Verification items for the finished model (mm, model axes). A direction names the side the tool comes from. Coordinates: 2 decimals unless noted, no trailing zeros. Order: outer loops, then holes, each group sorted by start corner. A loop starts at its lowest first (then second) coordinate and runs counter-clockwise, first axis right, second up. Notation, with made-up numbers: M 66,-34 L 94,-34 A23 ccw 94,-11 Z; hole C 5.5,-16 d11. An arc over 180 degrees is marked long. Return JSON: item names as keys, results as strings. Group by question number.
1. Section check D-D, the plane z = -4. Record the cut outline in (x, y).
2. Section check A-A, the plane y = 0.1. Record the cut outline in (x, z), plus the area to 3 significant figures.
3. Mould release check, pull along X, two halves, no side actions. Record for faces 1 (the flat face through (-45, 0, 9.5)), 2 (the flat face through (0, 0, 3)), 3 (the flat face through (-57.5, 0, 0)): +X half, -X half, draft (parallel to the pull), parting line (faces both ways), or undercut.
4. Section check C-C, the plane x = -6. Record the cut outline in (y, z).
5. Section check B-B, the plane z = 7.25. Record the cut outline in (x, y).
6. Material ranges on line 1 along X through (y, z) = (1.4, 5.75); line 2 along X through (y, z) = (-0.65, -6.5); line 3 along Z through (x, y) = (-10.5, 0.65), recorded low to high.
7. Set-up check for faces 4 (the cylindrical face through (25.617, -0.028, -8.294)), 5 (the cylindrical face through (-25.617, -0.028, 8.294)), 6 (the flat face through (-45, 0, -9.5)): record each of +Z, -Z, +X, -X, +Y, -Y from which the full face is reachable in a straight line by a thin tool's end or side.
```python
from build123d import *

# Parameters (mm, degrees)
F1_DEPTH = 2


with BuildPart() as f1:
    # F0 (on Front) → F1 (new body, symmetric)
    with BuildSketch(Plane.XZ):
        with BuildLine():
            Line((11.751494, 3), (0, 3))
            Line((0, 3), (-11.751494, 3))
            ThreePointArc((-11.751494, 3), (-15.797231, 3.597313), (-19.497744, 5.338285))
            ThreePointArc((-19.497744, 5.338285), (-25.709291, 8.323868), (-32.5, 9.5))
            Line((-32.5, 9.5), (-57.5, 9.5))
            Line((-57.5, 9.5), (-57.5, -9.5))
            Line((-57.5, -9.5), (-32.5, -9.5))
            ThreePointArc((-32.5, -9.5), (-25.709291, -8.323868), (-19.497744, -5.338285))
            ThreePointArc((-19.497744, -5.338285), (-15.797231, -3.597313), (-11.751494, -3))
            Line((-11.751494, -3), (0, -3))
            Line((0, -3), (11.751494, -3))
            ThreePointArc((11.751494, -3), (15.797231, -3.597313), (19.497744, -5.338285))
            ThreePointArc((19.497744, -5.338285), (25.709291, -8.323868), (32.5, -9.5))
            Line((32.5, -9.5), (57.5, -9.5))
            Line((57.5, -9.5), (57.5, 9.5))
            Line((57.5, 9.5), (32.5, 9.5))
            ThreePointArc((32.5, 9.5), (25.709291, 8.323868), (19.497744, 5.338285))
            ThreePointArc((19.497744, 5.338285), (15.797231, 3.597313), (11.751494, 3))
        make_face()
    extrude(amount=F1_DEPTH, both=True)


solid = f1.part
```
Answers follow:
{
 "1": {"outline": "M -57.5,-2 L -16.95,-2 L -16.95,2 L -57.5,2 Z; M 16.95,-2 L 57.5,-2 L 57.5,2 L 16.95,2 Z"},
 "2": {"outline": "M -57.5,-9.5 L -32.5,-9.5 A25 ccw -19.5,-5.34 A14 cw -11.75,-3 L 11.75,-3 A14 cw 19.5,-5.34 A25 ccw 32.5,-9.5 L 57.5,-9.5 L 57.5,9.5 L 32.5,9.5 A25 ccw 19.5,5.34 A14 cw 11.75,3 L -11.75,3 A14 cw -19.5,5.34 A25 ccw -32.5,9.5 L -57.5,9.5 Z", "area": "1,630 mm^2"},
 "3": {"face 1": "draft", "face 2": "undercut", "face 3": "-X half"},
 "4": {"outline": "M -2,-3 L 2,-3 L 2,3 L -2,3 Z"},
 "5": {"outline": "M -57.5,-2 L -22.93,-2 L -22.93,2 L -57.5,2 Z; M 22.93,-2 L 57.5,-2 L 57.5,2 L 22.93,2 Z"},
 "6": {"line 1": "-57.5 to -20.14, 20.14 to 57.5", "line 2": "-57.5 to -21.43, 21.43 to 57.5", "line 3": "-3 to 3"},
 "7": {"face 4": "-Z, +Y, -Y", "face 5": "+Z, +Y, -Y", "face 6": "-Z, +X, -X, +Y, -Y"}
}
